from build123d import *

# Parameters (mm, degrees)
F0_R      = 12.7
F1_DEPTH  = 12.319
F2_R      = 11.0109
F3_DEPTH  = 3.175
F5_DEPTH  = 33.02
F9_DEPTH  = 25.4
F10_DEPTH = 25.4


with BuildPart() as f1:
    # F0 (on Right) → F1 (new body)
    with BuildSketch(Plane.YZ):
        Circle(F0_R)
    extrude(amount=F1_DEPTH)

    # F2 (on face) → F3 (join)
    with BuildSketch(Plane(origin=(0, 0, 0), x_dir=(0, -1, 0), z_dir=(-1, 0, 0))):
        Circle(F2_R)
    extrude(amount=F3_DEPTH)

    # F4 (on face) → F5 (join)
    with BuildSketch(Plane(origin=(-3.175, 0, 0), x_dir=(0, -1, 0), z_dir=(-1, 0, 0))):
        with BuildLine():
            Line((-11.5951, 5.1810863716), (-11.5951, -5.1810863716))
            ThreePointArc((-11.5951, -5.1810863716), (0, -12.7), (11.5951, -5.1810863716))
            Line((11.5951, -5.1810863716), (11.5951, 5.1810863716))
            ThreePointArc((11.5951, 5.1810863716), (0, 12.7), (-11.5951, 5.1810863716))
        make_face()
    extrude(amount=F5_DEPTH)

    # F6 (on Front) → F7 (revolve)
    with BuildSketch(Plane.XZ):
        with BuildLine():
            Line((-36.195, 12.7), (-56.0844132237, 9.2605550421))
            ThreePointArc((-56.0844132237, 9.2605550421), (-61.6723144832, 6.0527812832), (-63.881, 0))
            Line((-63.881, 0), (-36.195, 0))
            Line((-36.195, 0), (-36.195, 12.7))
        make_face()
    revolve(axis=Axis((-50.038, 0, 0), (1, 0, 0)))

    # F8 (on face) → F9 (cut)
    with BuildSketch(Plane.YZ.offset(-36.195)):
        with BuildLine():
            Line((-11.5951, -5.1810863716), (-11.5951, 5.1810863716))
            ThreePointArc((-11.5951, 5.1810863716), (-12.7, 0), (-11.5951, -5.1810863716))
        make_face()
    extrude(amount=-F9_DEPTH, mode=Mode.SUBTRACT)

    # F10 (cut): a face of the model
    f10_faces = [f1.faces().sort_by_distance(p)[0] for p in [
        (-36.195, 12.0387504501, 0),
    ]]
    extrude(f10_faces, amount=-F10_DEPTH, mode=Mode.SUBTRACT)


solid = f1.part
Verification items for the finished model (mm, model axes). A direction names the side the tool comes from. Give positions to 0.01 mm unless a question says otherwise; leave off trailing zeros. Loops run counter-clockwise (first coordinate to the right, second up) from the corner with the lowest first, then second, coordinate; pieces in that order, holes last.
1. Cross-section at D-D on x = 1. Record the cut outline in (y, z).
Derived:
outline: circle Ø25.4 at (0, 0)
2. Release check for a two-part mould opening along X. For faces 5 (the cylindrical face through (-1.565, -5.919, 9.284)), 6 (the flat face through (0, -0.1, 11.3)), 7 (the cylindrical face through (6.07, -2.75, -12.4)), 8 (the conical face through (-48.49, 9.38, 4.88)) record: +X half, -X half, draft (parallel to the pull), parting line (faces both ways), or undercut.
Derived:
face 5: undercut
face 6: undercut
face 7: draft
face 8: -X half
3. Cross-section at A-A on z = 0. Record the cut outline in (x, y) (3 decimals).
Derived:
outline: (-56.084, -9.261) - (-42.584, -11.595) - (-3.175, -11.595) - (-3.175, -11.011) - (0, -11.011) - (0, -12.7) - (12.319, -12.7) - (12.319, 12.7) - (0, 12.7) - (0, 11.011) - (-3.175, 11.011) - (-3.175, 11.595) - (-42.584, 11.595) - (-56.084, 9.261) arc R9.398 ccw to start
4. Go/stop test with flat-tipped pins: P1, Ø8, axis at x = -2, y = -8.5, coming from the +Z side; P2, Ø4, axis at x = -1.5, y = 6, coming from the -Z side; P3, Ø2, axis at y = -2, z = -1.5, coming from the -X side. Record where each tip stops, or that it passes through.
Derived:
P1: stops at z = 11.81
P2: stops at z = -11.81
P3: stops at x = -63.76
5. Cross-section at B-B on y = 0. Record the cut outline in (x, z) (3 decimals).
Derived:
outline: (-56.084, -9.261) - (-36.195, -12.7) - (-3.175, -12.7) - (-3.175, -11.011) - (0, -11.011) - (0, -12.7) - (12.319, -12.7) - (12.319, 12.7) - (0, 12.7) - (0, 11.011) - (-3.175, 11.011) - (-3.175, 12.7) - (-36.195, 12.7) - (-56.084, 9.261) arc R9.398 ccw to start
6. Tool access check on faces 1 (the flat face through (-23, 11.595, 0)), 2 (the flat face through (-3.175, 10, 6)), 3 (the cylindrical face through (-19.5, 0.2, -12.7)), 4 (the flat face through (-23, -11.595, 0)). Record the directions out of +Z, -Z, +X, -X, +Y, -Y that give a thin tool (end or side, any length) a straight path to the whole face; none if there is none.
Derived:
face 1: +Z, -Z, -X, +Y
face 2: none
face 3: -Z, +X, -X
face 4: +Z, -Z, -X, -Y
7. Material ranges on probe 1 along Y at (x, z) = (-42.5, -0.25); probe 2 along Z at (x, y) = (-35.5, 0); probe 3 along Y at (x, z) = (-55.5, -6.25), recorded low to high.
Derived:
probe 1: y = -11.6 to 11.6
probe 2: z = -12.7 to 12.7
probe 3: y = -6.97 to 6.97
8. Cross-section at C-C on x = -19. Record the cut outline in (y, z), and give its area (3 significant figures).
Derived:
outline: (-11.6, -5.18) arc R12.7 ccw to (11.6, -5.18) - (11.6, 5.18) arc R12.7 ccw to (-11.6, 5.18) - close
area: 491 mm2
